from build123d import *

# Parameters (mm, degrees)
F0_W     = 67
F0_H     = 17
F1_DEPTH = 5
F2_DEPTH = 30
F3_DEPTH = 30


with BuildPart() as f1:
    # F0 (on Front) → F1 (new body)
    with BuildSketch(Plane.XZ):
        Rectangle(F0_W, F0_H)
        with BuildLine():
            ThreePointArc((-17.498445447, 0.1526953798), (-17.4988340953, 0.0763437334), (-17.5, 0))
            ThreePointArc((-17.5, 0), (-32.4980567986, 0.2290470263), (-17.498445447, 0.1526953798))
        make_face(mode=Mode.SUBTRACT)
        with BuildLine():
            ThreePointArc((-7.5, 0), (0, 7.5), (7.5, 0))
            ThreePointArc((7.5, 0), (0, -7.5), (-7.5, 0))
        make_face(mode=Mode.SUBTRACT)
        with BuildLine():
            ThreePointArc((32.4989989183, 0.1225366207), (25.0602692732, -7.3772131047), (17.5, 0))
            ThreePointArc((17.5, 0), (24.9377285633, 7.6222863461), (32.4989989183, 0.1225366207))
        make_face(mode=Mode.SUBTRACT)
    extrude(amount=F1_DEPTH)

    # F0 (on Front) → F2 (join)
    with BuildSketch(Plane.XZ):
        with BuildLine():
            ThreePointArc((-17.498445447, 0.1526953798), (-32.4980567986, 0.2290470263), (-17.5, 0))
            ThreePointArc((-17.5, 0), (-17.4988340953, 0.0763437334), (-17.498445447, 0.1526953798))
        make_face()
    extrude(amount=F2_DEPTH)

    # F0 (on Front) → F3 (join)
    with BuildSketch(Plane.XZ):
        with BuildLine():
            ThreePointArc((-7.5, 0), (0, -7.5), (7.5, 0))
            ThreePointArc((7.5, 0), (0, 7.5), (-7.5, 0))
        make_face()
        with BuildLine():
            ThreePointArc((32.4989989183, 0.1225366207), (24.9377285633, 7.6222863461), (17.5, 0))
            ThreePointArc((17.5, 0), (25.0602692732, -7.3772131047), (32.4989989183, 0.1225366207))
        make_face()
    extrude(amount=F3_DEPTH)


solid = f1.part
For this review, take the finished solid that the model builds, in its own axes (mm). A direction names the side the tool comes from. Round coordinates to 2 decimals unless told otherwise and drop trailing zeros. Loops run counter-clockwise (first coordinate to the right, second up) from the corner with the lowest first, then second, coordinate; pieces in that order, holes last. Notation, with made-up numbers: (-38, -23.75) - (-30, -23.75) arc R28 ccw to (-30, 15.25) - close; hole circle Ø9 at (31, 49.25). An arc over 180 degrees is marked (long way). Use one line per item in the form item = value.
Item 1: Consider section C-C on y = -19.25. Write out the cut boundary in (x, z), then the cut area to 3 significant figures.
Answers:
outline = circle Ø15 at (-25, 0.15); circle Ø15 at (0, 0); circle Ø15 at (25, 0.12)
area = 530 mm^2
Item 2: For line 1 (X direction, y = -9.75, z = -3.75); line 2 (X direction, y = -20, z = 4.5); line 3 (Y direction, x = 21, z = -6.75), list the stretches that pass through material, from the lowest coordinate up.
Answers:
line_1 = -31.4 to -18.59, -6.5 to 6.5, 18.58 to 31.42
line_2 = -31.11 to -18.89, -6 to 6, 18.91 to 31.09
line_3 = -5 to 0
Item 3: Consider section D-D on x = 10.5. Write out the cut boundary in (y, z), then the cut area to 3 significant figures.
Answers:
outline = (-5, -8.5) - (0, -8.5) - (0, 8.5) - (-5, 8.5) - close
area = 85.0 mm^2
Item 4: Consider section B-B on z = 5.25. Write out the cut boundary in (x, y), then the cut area to 3 significant figures.
Answers:
outline = (-33.5, -5) - (-30.5, -5) - (-30.5, -30) - (-19.5, -30) - (-19.5, -5) - (-5.36, -5) - (-5.36, -30) - (5.36, -30) - (5.36, -5) - (19.53, -5) - (19.53, -30) - (30.47, -30) - (30.47, -5) - (33.5, -5) - (33.5, 0) - (-33.5, 0) - close
area = 1,150 mm^2
Item 5: Consider section A-A on x = 0. Write out the cut boundary in (y, z).
Answers:
outline = (-30, -7.5) - (-5, -7.5) - (-5, -8.5) - (0, -8.5) - (0, 8.5) - (-5, 8.5) - (-5, 7.5) - (-30, 7.5) - close
Item 6: Mouldability with a two-part tool opening along X and no side actions: class faces 1 (the flat face through (0, -2, -8.5)), 2 (the cylindrical face through (-1.63, -17.32, -7.32)), 3 (the flat face through (-33.5, -2, 0)) as +X half, -X half, draft (parallel to the pull), parting line (faces both ways), or undercut.
Answers:
face_1 = draft
face_2 = undercut
face_3 = -X half
Item 7: Tool access review of faces 4 (the cylindrical face through (18.025, -17.325, 2.882)), 5 (the flat face through (0, 0, 0)): name each direction out of +Z, -Z, +X, -X, +Y, -Y from which nothing blocks a thin tool from reaching the whole face with its end or side.
Answers:
face_4 = -Y
face_5 = +Z, -Z, +X, -X, +Y
Item 8: Clearance check with flat-ended pins moving along their axes: P1, Ø3, axis at y = -21.5, z = -6.5, coming from the +X side; P2, Ø3, axis at x = 1, y = -20, coming from the -Z side; P3, Ø10, axis at y = -20.5, z = -3.5, coming from the -X side. State where each tip first meets the part, or that it passes through.
Answers:
P1 = 30.48
P2 = -7.5
P3 = -32.5
